Model file for the job. Use its own axes, mm. A direction names the side the tool comes from. Give positions to 0.01 mm unless a question says otherwise; leave off trailing zeros. Order: outer loops, then holes, each group sorted by start corner. A loop starts at its lowest first (then second) coordinate and runs counter-clockwise, first axis right, second up. Notation, with made-up numbers: M 56,81.25 L 108,81.25 A31 ccw 108,120.25 Z; hole C 53,-23.75 d8. An arc over 180 degrees is marked long. Return JSON: item names as keys, results as strings. Group by question number.
1. Slice it at B-B on x = 17.5. List the corners of the cut face in (y, z), then the cut area to 3 significant figures.
2. 3-axis set-ups, long thin cutter, end or side, ignore diameter. For faces 1 (the face through (48, 70, 9)), 2 (the face through (29, 9, 23)), 3 (the face through (59, 4, 16)): which of +Z, -Z, +X, -X, +Y, -Y reach the whole face in a straight line?
3. Wall check: probe 1 along Z at (x, y) = (46, 2.25); probe 2 along Y at (x, z) = (33, 31). Give the ranges that are in metal, low to high. Write a range as [from, to].
4. Slice it at D-D on y = 34.5. List the corners of the cut face in (x, z), then the cut area to 3 significant figures.
5. Two-plate mould, pull along Y, no slides. Class faces 4 (the face through (57.79, 57.48, 26.82)), 5 (the face through (64, 64, 27)), 6 (the face through (55.293, 4.437, 33.091)): released by +Y, released by -Y, zero draft, split by the parting line, or undercut.
6. Slice it at A-A on z = 15. List the corners of the cut face in (x, y), then the cut area to 3 significant figures.
7. Slice it at C-C on z = 36. List the corners of the cut face in (x, y).
8. Pin check, flat tips, straight feed: pin 1 (2 mm diameter, centred on x = 21, z = 16.5, fed in from +Y); pin 2 (10 mm diameter, centred on y = 56, z = 8, fed in from -X); pin 3 (10 mm diameter, centred on y = 3, z = 15, fed in from +X). Stop position of each tip, or through.
from build123d import *

# Parameters (mm, degrees)
F1_DEPTH = 9
F2_R     = 7
F3_DEPTH = 9
F4_R     = 5.5
F5_DEPTH = 9


with BuildPart() as f1:
    # F0 (on Top) → F1 (new body)
    with BuildSketch(Plane.XY):
        Polygon((52.686291501, 75.313708499), (0, 0), (59, 0), (75.313708499, 52.686291501), align=None)
    extrude(amount=F1_DEPTH)

    # F2 (on face) → F3 (join)
    with BuildSketch(Plane(origin=(64, 64, 0), x_dir=(-0.7071067812, 0.7071067812, 0), z_dir=(0.7071067812, 0.7071067812, 0))):
        with BuildLine():
            Line((-16, 38), (-16, 9))
            Line((-16, 9), (16, 9))
            Line((16, 9), (16, 38))
            ThreePointArc((16, 38), (0, 54), (-16, 38))
        make_face()
        with Locations((0, 38)):
            Circle(F2_R, mode=Mode.SUBTRACT)
    extrude(amount=-F3_DEPTH)

    # F4 (on face) → F5 (join)
    with BuildSketch(Plane.XZ):
        with BuildLine():
            Line((0, 24), (0, 9))
            Line((0, 9), (59, 9))
            Line((59, 9), (59, 24))
            ThreePointArc((59, 24), (55.1923881554, 33.1923881554), (46, 37))
            Line((46, 37), (13, 37))
            ThreePointArc((13, 37), (3.8076118446, 33.1923881554), (0, 24))
        make_face()
        with Locations((13, 24)):
            Circle(F4_R, mode=Mode.SUBTRACT)
        with Locations((46, 24)):
            Circle(F4_R, mode=Mode.SUBTRACT)
    extrude(amount=-F5_DEPTH)


solid = f1.part
Result:
{
 "1": {"outline": "M 0,0 L 25.02,0 L 25.02,9 L 9,9 L 9,20.84 L 0,20.84 Z; M 0,27.16 L 9,27.16 L 9,37 L 0,37 Z", "area": "420 mm2"},
 "2": {"face 1": "-Z, -X, +Y", "face 2": "+Z, +X, -X", "face 3": "+Z, +X, -Y"},
 "3": {"probe 1": "z = [0, 18.5], [29.5, 37]", "probe 2": "y = [0, 9]"},
 "4": {"outline": "M 24.13,0 L 69.68,0 L 69.68,9 L 24.13,9 Z", "area": "410 mm2"},
 "5": {"face 4": "undercut", "face 5": "released by +Y", "face 6": "zero draft"},
 "6": {"outline": "M 0,0 L 59,0 L 59,9 L 0,9 Z; M 46.32,68.95 L 68.95,46.32 L 75.31,52.69 L 52.69,75.31 Z", "area": "819 mm2"},
 "7": {"outline": "M 8,0 L 51,0 L 51,9 L 8,9 Z; M 46.32,68.95 L 52.89,62.38 L 59.26,68.74 L 52.69,75.31 Z; M 62.38,52.89 L 68.95,46.32 L 75.31,52.69 L 68.74,59.26 Z"},
 "8": {"pin 1": "stops at y = 9", "pin 2": "stops at x = 35.68", "pin 3": "stops at x = 59"}
}
